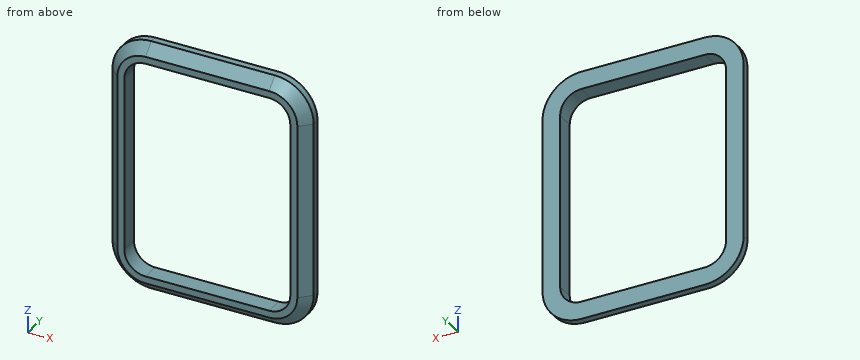
from build123d import *

# Parameters (mm, degrees)
F1_DEPTH = 5
F2_SIZE  = 3


with BuildPart() as f1:
    # F0 (on Front) → F1 (new body)
    with BuildSketch(Plane.XZ):
        with BuildLine():
            Line((17.307692, 36.088463), (-17.692308, 36.088463))
            ThreePointArc((-17.692308, 36.088463), (-25.470484, 32.866637), (-28.692309, 25.088462))
            Line((-28.692309, 25.088462), (-28.692309, -24.511538))
            ThreePointArc((-28.692309, -24.511538), (-25.470484, -32.289714), (-17.692308, -35.51154))
            Line((-17.692308, -35.51154), (17.307692, -35.51154))
            ThreePointArc((17.307692, -35.51154), (25.085868, -32.289714), (28.307693, -24.511538))
            Line((28.307693, -24.511538), (28.307693, 25.088462))
            ThreePointArc((28.307693, 25.088462), (25.085868, 32.866637), (17.307692, 36.088463))
        make_face()
        with BuildLine():
            ThreePointArc((-23.692308, 25.088462), (-21.934949, 29.331102), (-17.692308, 31.088462))
            Line((-17.692308, 31.088462), (17.307692, 31.088462))
            ThreePointArc((17.307692, 31.088462), (21.550333, 29.331102), (23.307692, 25.088462))
            Line((23.307692, 25.088462), (23.307692, -24.511538))
            ThreePointArc((23.307692, -24.511538), (21.550333, -28.754179), (17.307692, -30.511538))
            Line((17.307692, -30.511538), (-17.692308, -30.511538))
            ThreePointArc((-17.692308, -30.511538), (-21.934949, -28.754179), (-23.692308, -24.511538))
            Line((-23.692308, -24.511538), (-23.692308, 25.088462))
        make_face(mode=Mode.SUBTRACT)
    extrude(amount=F1_DEPTH)

    # F2
    f2_edges = [f1.edges().sort_by_distance(p)[0] for p in [
        (28.307693, -5, 0.288462),
    ]]
    chamfer(f2_edges, length=F2_SIZE)


solid = f1.part
Check sheet for the modelled part. Datum: model origin and axes. Units: mm. Coordinates: 2 decimals unless noted, no trailing zeros. Write each loop counter-clockwise with the first axis right and the second up, starting at its lowest first coordinate (ties: lowest second). Pieces come first, ordered by that corner, then holes. Notation, with made-up numbers: M 23.25,-26 L 63.25,-26 A24 ccw 63.25,-14 Z; hole C -39.5,-2.5 d1. An arc over 180 degrees is marked long. Answer as CSV lines item,"result".
Q1. Cross-section at B-B (x = 13). Record the boundary of the cut face in (y, z).
Check result:
outline,"M -5,-32.51 L -2,-35.51 L 0,-35.51 L 0,-30.51 L -5,-30.51 Z; M -5,31.09 L 0,31.09 L 0,36.09 L -2,36.09 L -5,33.09 Z"
Q2. Cross-section at C-C (y = -3.2). Record the boundary of the cut face in (x, z).
Check result:
outline,"M -27.49,-24.51 A9.8 ccw -17.69,-34.31 L 17.31,-34.31 A9.8 ccw 27.11,-24.51 L 27.11,25.09 A9.8 ccw 17.31,34.89 L -17.69,34.89 A9.8 ccw -27.49,25.09 Z; hole M -23.69,-24.51 A6 ccw -17.69,-30.51 L 17.31,-30.51 A6 ccw 23.31,-24.51 L 23.31,25.09 A6 ccw 17.31,31.09 L -17.69,31.09 A6 ccw -23.69,25.09 Z"
Q3. Go/stop test with flat-tipped pins: pin 1 (2.5 mm diameter, centred on x = 6, y = -3.5, fed in from +Z); pin 2 (2.5 mm diameter, centred on x = 2.5, y = -2.5, fed in from -Z). Record where each tip stops, or that it passes through.
Check result:
pin 1,"z = 35.84"
pin 2,"z = -35.51"
Q4. Material ranges on probe 1 along X at (y, z) = (-0.4, 7); probe 2 along Z at (x, y) = (-11, -1.4); probe 3 along X at (y, z) = (-2.1, -28), recorded low to high. Write a range as from..to.
Check result:
probe 1,"-28.69..-23.69, 23.31..28.31"
probe 2,"-35.51..-30.51, 31.09..36.09"
probe 3,"-28.02..-22.57, 22.19..27.63"
Q5. Cross-section at A-A (z = -9). Record the boundary of the cut face in (x, y), then the cut area to 3 significant figures.
Check result:
outline,"M -28.69,-2 L -25.69,-5 L -23.69,-5 L -23.69,0 L -28.69,0 Z; M 23.31,-5 L 25.31,-5 L 28.31,-2 L 28.31,0 L 23.31,0 Z"
area,"41.0 mm^2"
